```python
from build123d import *

# Parameters (mm, degrees)
F0_W      = 93
F0_H      = 15
F1_DEPTH  = 1.5
F2_W      = 1.5
F2_H      = 15
F3_DEPTH  = 14.3
F4_DEPTH  = 17.83
F6_DEPTH  = 10.5
F7_DEPTH  = 1.5
F8_R      = 1.5
F8_R_2    = 1.45
F9_DEPTH  = 90
F10_R     = 1.625
F11_DEPTH = 1.5


with BuildPart() as f1:
    # F0 (on Top) → F1 (new body)
    with BuildSketch(Plane.XY):
        with Locations((4.7561880201, -11.8954138505)):
            Rectangle(F0_W, F0_H)
    extrude(amount=F1_DEPTH)

    # F2 (on face) → F3 (join)
    with BuildSketch(Plane.XY.offset(1.5)):
        with Locations((-40.9938119799, -11.8954138505)):
            Rectangle(F2_W, F2_H)
    extrude(amount=F3_DEPTH)

    # F2 (on face) → F4 (join)
    with BuildSketch(Plane.XY.offset(1.5)):
        with Locations((50.5061880201, -11.8954138505)):
            Rectangle(F2_W, F2_H)
    extrude(amount=F4_DEPTH)

    # F5 (on face) → F6 (join)
    with BuildSketch(Plane.YZ.offset(51.2561880201)):
        with BuildLine():
            ThreePointArc((-19.3954138505, 11.83), (-11.8954138505, 4.33), (-4.3954138505, 11.83))
            ThreePointArc((-4.3954138505, 11.83), (-6.5921129916, 17.1333008589), (-11.8954138505, 19.33))
            ThreePointArc((-11.8954138505, 19.33), (-17.1987147094, 17.1333008589), (-19.3954138505, 11.83))
        make_face()
    extrude(amount=F6_DEPTH)

    # F7 (cut, through all): faces of the model
    f7_faces = [f1.faces().sort_by_distance(p)[0] for p in [
        (51.2561880201, -6.0706733926, 17.6547404579),
        (51.2561880201, -17.7201543084, 17.6547404579),
    ]]
    extrude(f7_faces, amount=-F7_DEPTH, mode=Mode.SUBTRACT)

    # F8 (on face) → F9 (join, through all)
    with BuildSketch(Plane(origin=(49.7561880201, 0, 0), x_dir=(0, -1, 0), z_dir=(-1, 0, 0))):
        with Locations((6.8954138505, 6.5)):
            Circle(F8_R)
        with Locations((11.8954138505, 11.83)):
            Circle(F8_R_2)
        with Locations((16.8954138505, 6.5)):
            Circle(F8_R)
    extrude(amount=F9_DEPTH)

    # F10 (on face) → F11 (cut, through all)
    with BuildSketch(Plane(origin=(0, 0, 0), x_dir=(1, 0, 0), z_dir=(0, 0, -1))):
        with Locations((-19.1188119799, 15.2704138505)):
            Circle(F10_R)
        with Locations((-19.1188119799, 8.5204138505)):
            Circle(F10_R)
        with Locations((29.1311880201, 8.5204138505)):
            Circle(F10_R)
        with Locations((29.1311880201, 15.2704138505)):
            Circle(F10_R)
    extrude(amount=-F11_DEPTH, mode=Mode.SUBTRACT)


solid = f1.part
```
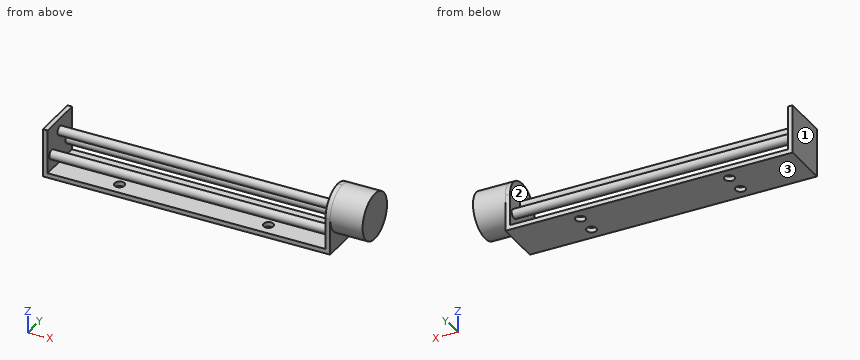
Verification items for the finished model (mm, model axes). Face numbers are marked on the shaded views. Coordinates: 2 decimals unless noted, no trailing zeros. Write each loop counter-clockwise with the first axis right and the second up, starting at its lowest first coordinate (ties: lowest second). Pieces come first, ordered by that corner, then holes. Notation, with made-up numbers: M 21.5,14.25 L 28.5,14.25 A13 cw 28.5,30.25 Z; hole C 3.25,-30.75 d8. An arc over 180 degrees is marked long. Answer as a JSON object with one key per item and string values. Group by question number.
(1) Cross-section at B-B, the plane z = 9.5. Record the cut outline in (x, y), and give its area (3 significant figures).
(2) Release check for a two-part mould opening along Z. For the marked faces 1, 2 and 3 record: +Z half, -Z half, draft (parallel to the pull), parting line (faces both ways), or undercut.
(3) Cross-section at A-A, the plane x = 46. Record the cut outline in (y, z).
(4) Material ranges on line 1 (X direction, y = -12.25, z = 1.75); line 2 (X direction, y = -7.25, z = 1); line 3 (X direction, y = -15, z = 12.75), recorded low to high.
(5) Gauge pin test, flat ends, axial feed: pin 1 (3 mm diameter, centred on x = 29.13, y = -15.27, fed in from -Z); pin 2 (1.9 mm diameter, centred on x = -19.12, y = -15.27, fed in from -Z); pin 3 (1.6 mm diameter, centred on x = -41, y = -8.5, fed in from +Z). Record the tip position at first contact, or that the pin passes through.
Reply:
{
 "1": {"outline": "M -41.74,-19.4 L -40.24,-19.4 L -40.24,-4.4 L -41.74,-4.4 Z; M 49.76,-19.4 L 51.26,-19.4 L 51.26,-19.02 L 61.76,-19.02 L 61.76,-4.77 L 51.26,-4.77 L 51.26,-4.4 L 49.76,-4.4 Z", "area": "195 mm²"},
 "2": {"face 1": "draft", "face 2": "undercut", "face 3": "-Z half"},
 "3": {"outline": "M -19.4,0 L -4.4,0 L -4.4,1.5 L -19.4,1.5 Z; C -16.9,6.5 d3; C -11.9,11.83 d2.9; C -6.9,6.5 d3"},
 "4": {"line 1": "-41.74 to -40.24, 49.76 to 51.26", "line 2": "-41.74 to -20.13, -18.11 to 28.12, 30.14 to 51.26", "line 3": "-41.74 to -40.24, 49.76 to 61.76"},
 "5": {"pin 1": "z = 5.01", "pin 2": "z = 5.16", "pin 3": "z = 15.8"}
}
